Design review of the part built by this model. Coordinates are the model's own, in mm. A direction names the side the tool comes from. Coordinates: 2 decimals unless noted, no trailing zeros. Loops run counter-clockwise (first coordinate to the right, second up) from the corner with the lowest first, then second, coordinate; pieces in that order, holes last. Notation, with made-up numbers: (82, 35) - (91, 35) arc R13 cw to (91, 51) - close; hole circle Ø2 at (3, -18.75). An arc over 180 degrees is marked (long way). Use one line per item in the form item = value. Start each with the question number.
(1) Add section A-A (x = 0). State the section outline as (y, z) points.
(2) Add section B-B (z = 36.5). State the section outline as (x, y) points.
(3) For L1, parallel to Z at x = 15.5, y = 61; L2, parallel to Z at x = 15.5, y = 55.1; L3, parallel to X at y = 57.5, z = 36.5, list the stretches that pass through material, from the lowest coordinate up.
(4) The part is to be moulded in two halves that separate along Z. For faces 1 (the face through (14.3, 59.3, 37.4)), 2 (the face through (0, 58, 42)), 3 (the face through (-14, 55.771, 35)), 4 (the face through (6, 52.771, 11)), say which applies: pulls with the +Z half, pulls with the -Z half, needs draft (parallel to the pull), parting line crosses it, or undercut.
(5) Clearance check with flat-ended pins moving along their axes: pin 1 Ø4.5 at (x, z) = (-15.5, 36) entering from -Y; pin 2 Ø3 at (x, z) = (16, 4) entering from -Y. State where each tip first meets the part, or that it passes through.
(6) Tool access review of faces 5 (the face through (-30, 58, 21)), 6 (the face through (17, 55.771, 4)): name each direction out of +Z, -Z, +X, -X, +Y, -Y from which nothing blocks a thin tool from reaching the whole face with its end or side.
(7) Add section D-D (z = 22). State the section outline as (x, y) points.
(8) Add section C-C (y = 61). State the section outline as (x, z) points, plus the area to 3 significant figures.
```python
from build123d import *

# Parameters (mm, degrees)
SKETCH1_W           = 60
SKETCH1_H           = 10
BOSS_EXTRUDE1_DEPTH = 42
SKETCH2_R           = 11
SKETCH2_R_2         = 1.5
CUT_EXTRUDE1_DEPTH  = 11
SKETCH3_R           = 2.85
CUT_EXTRUDE2_DEPTH  = 3


with BuildPart() as part:
    # Sketch1 → Boss-Extrude1 (new body)
    with BuildSketch(Plane.XY):
        with Locations((0, 57.771455045)):
            Rectangle(SKETCH1_W, SKETCH1_H)
    extrude(amount=BOSS_EXTRUDE1_DEPTH)

    # Sketch2 → Cut-Extrude1 (cut, through all)
    with BuildSketch(Plane(origin=(0, 62.771455045, 0), x_dir=(1, 0, 0), z_dir=(0, 1, 0))):
        with Locations((0, -21)):
            Circle(SKETCH2_R)
        with Locations((-15.5, -36.5)):
            Circle(SKETCH2_R_2)
        with Locations((15.5, -36.5)):
            Circle(SKETCH2_R_2)
        with Locations((-15.5, -5.5)):
            Circle(SKETCH2_R_2)
        with Locations((15.5, -5.5)):
            Circle(SKETCH2_R_2)
    extrude(amount=-CUT_EXTRUDE1_DEPTH, mode=Mode.SUBTRACT)

    # Sketch3 → Cut-Extrude2 (cut)
    with BuildSketch(Plane.XZ.offset(-52.771455045)):
        with Locations((-15.5, 36.5)):
            Circle(SKETCH3_R)
        with Locations((15.5, 36.5)):
            Circle(SKETCH3_R)
        with Locations((15.5, 5.5)):
            Circle(SKETCH3_R)
        with Locations((-15.5, 5.5)):
            Circle(SKETCH3_R)
    extrude(amount=-CUT_EXTRUDE2_DEPTH, mode=Mode.SUBTRACT)


solid = part.part
```
Computed values:
q1.outline = (52.77, 0) - (62.77, 0) - (62.77, 10) - (52.77, 10) - close; (52.77, 32) - (62.77, 32) - (62.77, 42) - (52.77, 42) - close
q2.outline = (-30, 52.77) - (-18.35, 52.77) - (-18.35, 55.77) - (-17, 55.77) - (-17, 62.77) - (-30, 62.77) - close; (-14, 55.77) - (-12.65, 55.77) - (-12.65, 52.77) - (12.65, 52.77) - (12.65, 55.77) - (14, 55.77) - (14, 62.77) - (-14, 62.77) - close; (17, 55.77) - (18.35, 55.77) - (18.35, 52.77) - (30, 52.77) - (30, 62.77) - (17, 62.77) - close
q3.L1 = 0 to 4, 7 to 35, 38 to 42
q3.L2 = 0 to 2.65, 8.35 to 33.65, 39.35 to 42
q3.L3 = -30 to -17, -14 to 14, 17 to 30
q4.face_1 = undercut
q4.face_2 = pulls with the +Z half
q4.face_3 = undercut
q4.face_4 = needs draft
q5.pin_1 = 55.77
q5.pin_2 = 52.77
q6.face_5 = +Z, -Z, -X, +Y, -Y
q6.face_6 = -Y
q7.outline = (-30, 52.77) - (-10.95, 52.77) - (-10.95, 62.77) - (-30, 62.77) - close; (10.95, 52.77) - (30, 52.77) - (30, 62.77) - (10.95, 62.77) - close
q8.outline = (-30, 0) - (30, 0) - (30, 42) - (-30, 42) - close; hole circle Ø3 at (-15.5, 5.5); hole circle Ø3 at (-15.5, 36.5); hole circle Ø22 at (0, 21); hole circle Ø3 at (15.5, 5.5); hole circle Ø3 at (15.5, 36.5)
q8.area = 2,110 mm^2
